Check sheet for the modelled part. Datum: model origin and axes. Units: mm. Face numbers are marked on the shaded views. A direction names the side the tool comes from. Give positions to 0.01 mm unless a question says otherwise; leave off trailing zeros. Order: outer loops, then holes, each group sorted by start corner. A loop starts at its lowest first (then second) coordinate and runs counter-clockwise, first axis right, second up.
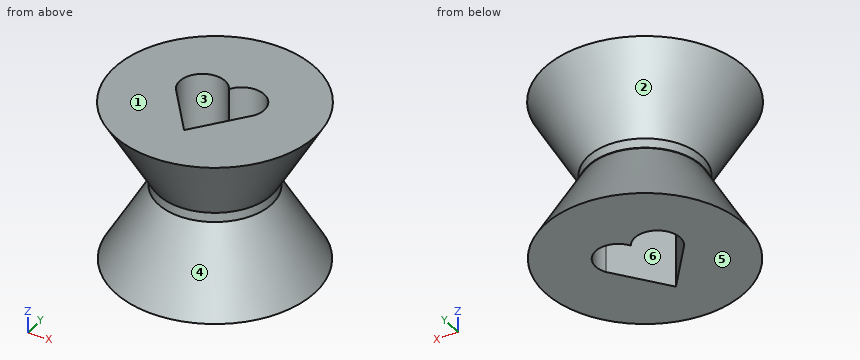
```python
from build123d import *

# Parameters (mm, degrees)
F0_R     = 38.1
F1_DEPTH = 50.8
F1_TAPER = -30
F2_DEPTH = 6.35
F3_R     = 37.6838107833
F4_DEPTH = 50.8
F4_TAPER = -30
F6_DEPTH = 127


with BuildPart() as f1:
    # F0 (on Top) → F1 (new body)
    with BuildSketch(Plane.XY):
        Circle(F0_R)
    extrude(amount=F1_DEPTH, taper=F1_TAPER)

    # F0 (on Top) → F2 (join)
    with BuildSketch(Plane.XY):
        Circle(F0_R)
    extrude(amount=-F2_DEPTH)

    # F3 (on face) → F4 (join)
    with BuildSketch(Plane(origin=(0, 0, -6.35), x_dir=(1, 0, 0), z_dir=(0, 0, -1))):
        Circle(F3_R)
    extrude(amount=F4_DEPTH, taper=F4_TAPER)

    # F5 (on face) → F6 (cut)
    with BuildSketch(Plane.XY.offset(50.8)):
        with BuildLine():
            Line((-26.2908060104, 0), (0, -33.7482951581))
            Line((0, -33.7482951581), (26.2908060104, 0))
            ThreePointArc((26.2908060104, 0), (20.8795288063, 20.8795288063), (0, 15.4682516023))
            ThreePointArc((0, 15.4682516023), (-20.8795288063, 20.8795288063), (-26.2908060104, 0))
        make_face()
    extrude(amount=-F6_DEPTH, mode=Mode.SUBTRACT)


solid = f1.part
```
Q1. Tool access check on the marked faces 4, 5 and 6. Record the directions out of +Z, -Z, +X, -X, +Y, -Y that give a thin tool (end or side, any length) a straight path to the whole face; none if there is none.
Q2. Sectioned sample at A-A, the plane z = 12. Record the cut outline in (x, y), plus the area to 3 significant figures.
Q3. Material ranges on line 1 (Y direction, x = 26, z = 14); line 2 (Z direction, x = 44, y = 1.5); line 3 (Z direction, x = -53, y = 20.5), recorded low to high.
Q4. Draft check along X on the marked faces 1, 2 and 3. Enter one of: pulls with the +X half, pulls with the -X half, needs draft (parallel to the pull), parting line crosses it, or undercut.
Q5. Go/stop test with flat-tipped pins: P1, Ø5, axis at x = -34.5, z = -29.5, coming from the +Y side; P2, Ø6, axis at y = 6, z = -35.5, coming from the -X side; P3, Ø3, axis at x = -1, z = 27.5, coming from the -Y side. Record where each tip stops, or that it passes through.
Q6. Sectioned sample at B-B, the plane z = -50. Record the cut outline in (x, y).
Filled in:
1. face 4: none
1. face 5: -Z, +X, -X, +Y, -Y
1. face 6: +Z, -Z
2. outline: circle Ø90.06 at (0, 0); hole (-26.29, 0) - (0, -33.75) - (26.29, 0) arc R15.25 ccw to (0, 15.47) arc R15.25 ccw to start
2. area: 4,340 mm2
3. line 1: y = -38.17 to -0.37, 15.94 to 38.17
3. line 2: z = -57.15 to -17.33, 10.26 to 50.8
3. line 3: z = -57.15 to -39.51, 32.44 to 50.8
4. face 1: needs draft
4. face 2: parting line crosses it
4. face 3: undercut
5. P1: stops at y = 40.5
5. P2: stops at x = -55.95
5. P3: stops at y = -54.83
6. outline: circle Ø125.77 at (0, 0); hole (-26.29, 0) - (0, -33.75) - (26.29, 0) arc R15.25 ccw to (0, 15.47) arc R15.25 ccw to start
